Part model, mm, in its own coordinate system. Face numbers are marked on the shaded views. A direction names the side the tool comes from. Round coordinates to 2 decimals unless told otherwise and drop trailing zeros. Loops run counter-clockwise (first coordinate to the right, second up) from the corner with the lowest first, then second, coordinate; pieces in that order, holes last. Notation, with made-up numbers: M 35.5,82.25 L 59.5,82.25 A32 cw 59.5,115.25 Z; hole C -11.75,-15 d3. An arc over 180 degrees is marked long. Put each result on its own line as item: value. Start each with the question number.
1) Drop flat-ended pins along their axis: pin 1 Ø3 at (x, z) = (1.5, 18.5) entering from +Y; pin 2 Ø3 at (x, y) = (-4.5, 85) entering from -Z; pin 3 Ø1 at (y, z) = (87, 42) entering from +X; pin 4 Ø6 at (y, z) = (87, 51.5) entering from -X. Give the stop position or say it passes through.
2) Slice it at C-C on x = 5. Give the cut face in (y, z).
3) Pull direction X, two halves, no side cores. Call the marked faces 1, 2, 3 and 4: +X half, -X half, draft (parallel to the pull), parting line (faces both ways), or undercut.
4) Slice it at D-D on x = -11.5. Give the cut face in (y, z), then the cut area to 3 significant figures.
5) Probe line 1 along Y through (x, z) = (0, 41); line 2 along X through (y, z) = (86.5, 29.5); line 3 along X through (y, z) = (87, 52). List the from-to ranges inside material, lowest first.
6) Which spindle directions (+Z, -Z, +X, -X, +Y, -Y) get a long thin tool onto all of the face, cutting with end or side? Do the marked faces 5, 6 and 7. Say none if no direction does.
7) Slice it at A-A on y = 84. Give the cut face in (x, z).
```python
from build123d import *

# Parameters (mm, degrees)
BOSS_EXTRUDE2_DEPTH = 67.5


with BuildPart() as part:
    # Sketch1 → Boss-Extrude2 (new body)
    with BuildSketch(Plane.XY):
        with BuildLine():
            Line((-17.624839098, 90.556097537), (-17.081964944, 88.53006361))
            ThreePointArc((-17.081964944, 88.53006361), (-17.06872461, 88.444180172), (-17.07434408, 88.357464009))
            Line((-17.07434408, 88.357464009), (-17.406101009, 86.465100374))
            ThreePointArc((-17.406101009, 86.465100374), (-17.408194108, 86.4114937), (-17.395962494, 86.359259189))
            Line((-17.395962494, 86.359259189), (-15.714560006, 81.953100992))
            ThreePointArc((-15.714560006, 81.953100992), (-15.62787368, 81.851299803), (-15.496416031, 81.826868517))
            Line((-15.496416031, 81.826868517), (-10.495838808, 82.618882142))
            ThreePointArc((-10.495838808, 82.618882142), (-10.378300643, 82.682811793), (-10.327369953, 82.806538448))
            Line((-10.327369953, 82.806538448), (-10.101894168, 87.364622968))
            ThreePointArc((-10.101894168, 87.364622968), (-10.0050052, 87.606431661), (-9.779768503, 87.737303149))
            ThreePointArc((-9.779768503, 87.737303149), (0.009655574, 88.693275712), (9.799075243, 87.737258013))
            ThreePointArc((9.799075243, 87.737258013), (10.024185058, 87.606531513), (10.121179929, 87.364961975))
            Line((10.121179929, 87.364961975), (10.351109341, 82.805609758))
            ThreePointArc((10.351109341, 82.805609758), (10.40209464, 82.682003526), (10.519568611, 82.618145345))
            Line((10.519568611, 82.618145345), (15.520145834, 81.82613172))
            ThreePointArc((15.520145834, 81.82613172), (15.65168662, 81.850611141), (15.738358224, 81.952543733))
            Line((15.738358224, 81.952543733), (17.415135527, 86.359286022))
            ThreePointArc((17.415135527, 86.359286022), (17.427307864, 86.411436625), (17.425205627, 86.464947668))
            Line((17.425205627, 86.464947668), (17.093421927, 88.357464009))
            ThreePointArc((17.093421927, 88.357464009), (17.087802457, 88.444180172), (17.101042791, 88.53006361))
            Line((17.101042791, 88.53006361), (17.643916946, 90.556097537))
            ThreePointArc((17.643916946, 90.556097537), (17.617025703, 90.718975393), (17.476837019, 90.806150319))
            Line((17.476837019, 90.806150319), (6.615644162, 92.236053485))
            ThreePointArc((6.615644162, 92.236053485), (6.457669761, 92.188132474), (6.389538924, 92.037764513))
            Line((6.389538924, 92.037764513), (6.389538924, 90.07390614))
            ThreePointArc((6.389538924, 90.07390614), (6.301670958, 89.861774106), (6.089538924, 89.77390614))
            Line((6.089538924, 89.77390614), (-6.570461076, 89.77390614))
            ThreePointArc((-6.570461076, 89.77390614), (-6.782593111, 89.861774106), (-6.870461076, 90.07390614))
            Line((-6.870461076, 90.07390614), (-6.870461076, 91.971938264))
            ThreePointArc((-6.870461076, 91.971938264), (-6.938591913, 92.122306225), (-7.096566315, 92.170227236))
            Line((-7.096566315, 92.170227236), (-17.457759172, 90.806150319))
            ThreePointArc((-17.457759172, 90.806150319), (-17.597947856, 90.718975393), (-17.624839098, 90.556097537))
        make_face()
    extrude(amount=BOSS_EXTRUDE2_DEPTH)


solid = part.part
```
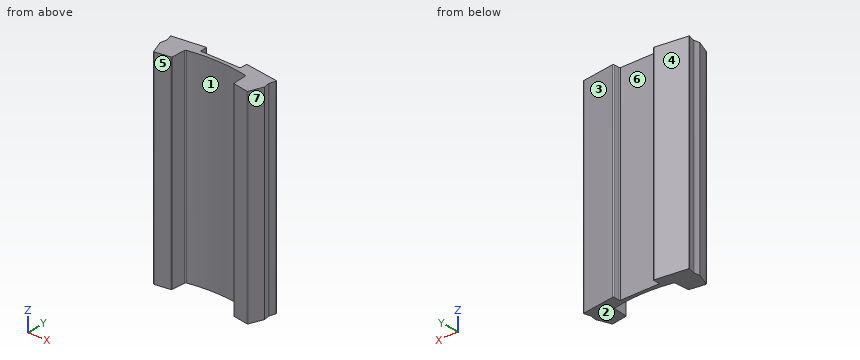
Recorded:
1. pin 1: stops at y = 89.77
1. pin 2: passes through
1. pin 3: stops at x = 17.42
1. pin 4: stops at x = -17.48
2. outline: M 88.45,0 L 89.77,0 L 89.77,67.5 L 88.45,67.5 Z
3. face 1: undercut
3. face 2: draft
3. face 3: +X half
3. face 4: -X half
4. outline: M 82.46,0 L 91.59,0 L 91.59,67.5 L 82.46,67.5 Z
4. area: 616 mm2
5. line 1: y = 88.69 to 89.77
5. line 2: x = -17.4 to -10.14, 10.16 to 17.42
5. line 3: x = -17.31 to -10.12, 10.14 to 17.33
6. face 5: +Z, -Z, -Y
6. face 6: +Z, -Z, +Y
6. face 7: +Z, -Z, +X, -Y
7. outline: M -16.5,0 L -10.27,0 L -10.27,67.5 L -16.5,67.5 Z; M 10.29,0 L 16.52,0 L 16.52,67.5 L 10.29,67.5 Z
